from build123d import *

# Parameters (mm, degrees)
ESQUISSE1_R             = 77.9
ESQUISSE1_R_2           = 2.25
ESQUISSE1_R_3           = 68.5
BOSS_EXTRU_1_DEPTH      = 13
ESQUISSE2_R             = 82.9
ESQUISSE2_R_2           = 77.9
BOSS_EXTRU_2_DEPTH      = 2
BOSS_EXTRU_2_DEPTH_BACK = 15


with BuildPart() as part:
    # Esquisse1 → Boss.-Extru.1 (new body)
    with BuildSketch(Plane.XY):
        Circle(ESQUISSE1_R)
        with Locations((0, 72.5)):
            Circle(ESQUISSE1_R_2, mode=Mode.SUBTRACT)
        with Locations((72.5, 0)):
            Circle(ESQUISSE1_R_2, mode=Mode.SUBTRACT)
        with Locations((0, -72.5)):
            Circle(ESQUISSE1_R_2, mode=Mode.SUBTRACT)
        with Locations((-72.5, 0)):
            Circle(ESQUISSE1_R_2, mode=Mode.SUBTRACT)
        Circle(ESQUISSE1_R_3, mode=Mode.SUBTRACT)
    extrude(amount=BOSS_EXTRU_1_DEPTH)

    # Esquisse2 → Boss.-Extru.2 (add, two sides)
    with BuildSketch(Plane.XY.offset(13)) as boss_extru_2_sk:
        Circle(ESQUISSE2_R)
        Circle(ESQUISSE2_R_2, mode=Mode.SUBTRACT)
    extrude(amount=BOSS_EXTRU_2_DEPTH)
    extrude(boss_extru_2_sk.sketch, amount=-BOSS_EXTRU_2_DEPTH_BACK)


solid = part.part
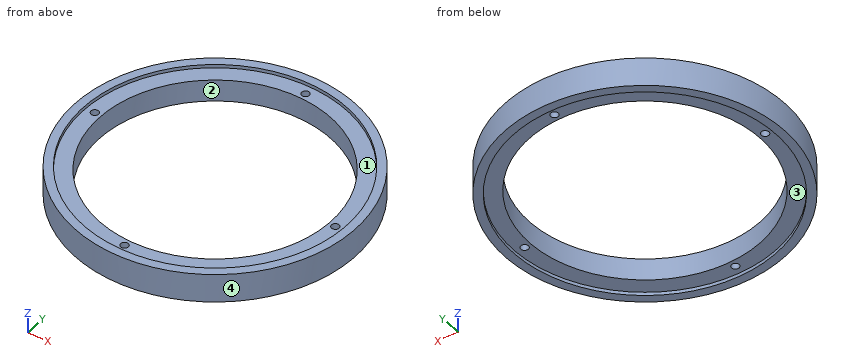
For this review, take the finished solid that the model builds, in its own axes (mm). Face numbers are marked on the shaded views. A direction names the side the tool comes from. Round coordinates to 2 decimals unless told otherwise and drop trailing zeros. Loops run counter-clockwise (first coordinate to the right, second up) from the corner with the lowest first, then second, coordinate; pieces in that order, holes last. Notation, with made-up numbers: (34, 64) - (42, 64) arc R37 ccw to (42, 103) - close; hole circle Ø10 at (45.5, 47.25). An arc over 180 degrees is marked (long way). Put each result on its own line as item: value. Start each with the question number.
1. Insertion check: P1, Ø7, axis at x = 72.5, y = 0, coming from the +Z side; P2, Ø3, axis at x = 18.5, z = 7.5, coming from the +Y side; P3, Ø3, axis at x = 37, z = 4, coming from the -Y side. Each pin has a flat end and moves straight along its axis. Give the tip position at first contact, or say it passes through.
2. Consider section C-C on y = -48.5. State the section outline as (x, z) points, plus the area to 3 significant figures.
3. For the marked faces 1 and 2, list the 3-axis set-ups (+Z, -Z, +X, -X, +Y, -Y) from which the entire face can be reached by the end or side of a thin tool; tool diameter is ignored.
4. Consider section D-D on x = -72.5. State the section outline as (y, z) points, plus the area to 3 significant figures.
5. Consider section B-B on z = 9. State the section outline as (x, y) points.
6. Mouldability with a two-part tool opening along Y and no side actions: class the marked faces 3 and 4 as +Y half, -Y half, draft (parallel to the pull), parting line (faces both ways), or undercut.
7. For probe 1 along Y at (x, z) = (0, 7); probe 2 along Y at (x, z) = (0, 14.5); probe 3 along X at (y, z) = (40, 13.75), list the stretches that pass through material, from the lowest coordinate up. Write a range as [from, to].
8. Consider section A-A on x = 0. State the section outline as (y, z) points, plus the area to 3 significant figures.
Result sheet:
1. P1: z = 13
1. P2: y = 81.14
1. P3: y = -74.91
2. outline: (-67.23, -2) - (-60.96, -2) - (-60.96, 0) - (-48.37, 0) - (-48.37, 13) - (-60.96, 13) - (-60.96, 15) - (-67.23, 15) - close; (48.37, 0) - (60.96, 0) - (60.96, -2) - (67.23, -2) - (67.23, 15) - (60.96, 15) - (60.96, 13) - (48.37, 13) - close
2. area: 540 mm^2
3. face 1: +Z
3. face 2: +Z, -Z
4. outline: (-40.2, -2) - (-28.5, -2) - (-28.5, 0) - (-2.25, 0) - (-2.25, 13) - (-28.5, 13) - (-28.5, 15) - (-40.2, 15) - close; (2.25, 0) - (28.5, 0) - (28.5, -2) - (40.2, -2) - (40.2, 15) - (28.5, 15) - (28.5, 13) - (2.25, 13) - close
4. area: 1,080 mm^2
5. outline: circle Ø165.8 at (0, 0); hole circle Ø4.5 at (-72.5, 0); hole circle Ø137 at (0, 0); hole circle Ø4.5 at (0, -72.5); hole circle Ø4.5 at (0, 72.5); hole circle Ø4.5 at (72.5, 0)
6. face 3: undercut
6. face 4: parting line
7. probe 1: [-82.9, -74.75], [-70.25, -68.5], [68.5, 70.25], [74.75, 82.9]
7. probe 2: [-82.9, -77.9], [77.9, 82.9]
7. probe 3: [-72.61, -66.85], [66.85, 72.61]
8. outline: (-82.9, -2) - (-77.9, -2) - (-77.9, 0) - (-74.75, 0) - (-74.75, 13) - (-77.9, 13) - (-77.9, 15) - (-82.9, 15) - close; (-70.25, 0) - (-68.5, 0) - (-68.5, 13) - (-70.25, 13) - close; (68.5, 0) - (70.25, 0) - (70.25, 13) - (68.5, 13) - close; (74.75, 0) - (77.9, 0) - (77.9, -2) - (82.9, -2) - (82.9, 15) - (77.9, 15) - (77.9, 13) - (74.75, 13) - close
8. area: 297 mm^2
